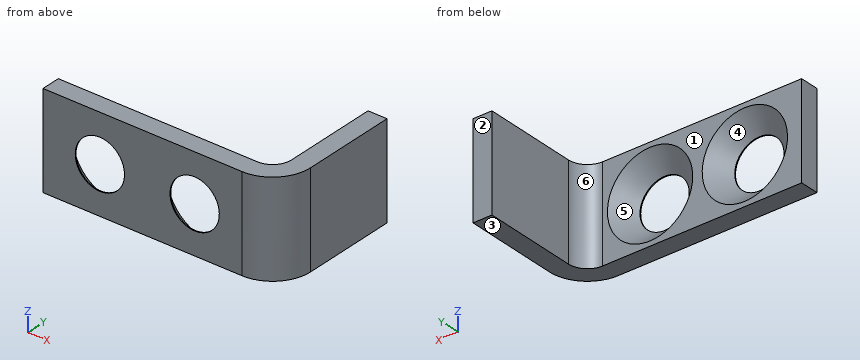
```python
from build123d import *

# Parameters (mm, degrees)
BASE_FLANGE1_DEPTH                          = 5
CSK_FOR_M2_CROSS_RECESSED_CTSK_HEAD_2_COUNT = 2
CSK_FOR_M2_CROSS_RECESSED_CTSK_HEAD_2_PITCH = 5


# Sheet-metal steps are written as plain solids
with BuildPart() as part:
    # Sketch1 → Base-Flange1 (new body)
    with BuildSketch(Plane.XY):
        with BuildLine():
            Line((-11.5, 0), (-1, 0))
            ThreePointArc((-1, 0), (-0.292893219, 0.292893219), (0, 1))
            Line((0, 1), (0, 6))
            Line((0, 6), (1, 6))
            Line((1, 6), (1, 1))
            ThreePointArc((1, 1), (0.414213562, -0.414213562), (-1, -1))
            Line((-1, -1), (-11.5, -1))
            Line((-11.5, -1), (-11.5, 0))
        make_face()
    extrude(amount=BASE_FLANGE1_DEPTH)

    # Sketch3 → CSK for M2 Cross recessed CTSK head wood screws1 (revolve, cut)
    with BuildSketch(Plane(origin=(-8.5, 0, 2.5), x_dir=(0, 0, 1), z_dir=(1, 0, 0))):
        Polygon((0, 0), (0, 1), (1.3, 1), (1.3, 0.95), (2.25, 0), align=None)
    csk_for_m2_cross_recessed_ctsk_head_wood = revolve(axis=Axis((-8.5, 6.35, 2.5), (0, -1, 0)), mode=Mode.SUBTRACT)

    # CSK for M2 Cross recessed CTSK head  2: CSK for M2 Cross recessed CTSK head wood screws1 ×2
    with Locations(*[(i * CSK_FOR_M2_CROSS_RECESSED_CTSK_HEAD_2_PITCH, 0, 0) for i in range(1, CSK_FOR_M2_CROSS_RECESSED_CTSK_HEAD_2_COUNT)]):
        add(csk_for_m2_cross_recessed_ctsk_head_wood, mode=Mode.SUBTRACT)


solid = part.part
```
The listing builds one solid part. Answer for the finished solid, in the listing's coordinates (mm). Face numbers are marked on the shaded views. A direction names the side the tool comes from. Give positions to 0.01 mm unless a question says otherwise; leave off trailing zeros. Loops run counter-clockwise (first coordinate to the right, second up) from the corner with the lowest first, then second, coordinate; pieces in that order, holes last. Notation, with made-up numbers: (24, 32) - (62, 32) arc R10 ccw to (62, 51) - close; hole circle Ø4 at (-29, 78.25). An arc over 180 degrees is marked (long way). Return JSON: item names as keys, results as strings. Group by question number.
1. Which of the six approach directions +Z, -Z, +X, -X, +Y, -Y give full straight-line access (tool end or side, diameter ignored) to the marked faces 1 and 2?
2. Straight lines are drawn through the part: line 1 (Y direction, x = -2.25, z = 0.4); line 2 (X direction, y = 1.5, z = 1.7); line 3 (Z direction, x = -9.5, y = -0.5). For each, find the intervals that lie inside material, in ascending order. Write a range as [from, to].
3. Find section B-B (y = -0.5). Write down the section's boundary in (x, z).
4. Find section C-C (z = 2.55). State how many separate pieces and enclosed holes the cut face has, then the cut area to 3 significant figures.
5. Find section A-A (x = -3.5). Write down the section's boundary in (y, z).
6. Determine the mould class of the marked faces 3, 4, 5 and 6 for opening direction Z: pulls with the +Z half, pulls with the -Z half, needs draft (parallel to the pull), parting line crosses it, or undercut.
7. Given pin 1 Ø2 at (y, z) = (2.5, 3.5) entering from -X; pin 2 Ø1.6 at (x, z) = (-8.5, 2.5) entering from -Y, each flat-ended and moving along its own axis, determine where each tip first touches the part or whether it passes through.
8. Find section D-D (y = 5.5). Write down the section's boundary in (x, z).
Verdict:
{
 "1": {"face 1": "+Z, -Z, -X, +Y", "face 2": "+Z, -Z, +X, -X, +Y"},
 "2": {"line 1": "y = [-1, 0]", "line 2": "x = [0, 1]", "line 3": "z = [0, 1.06], [3.94, 5]"},
 "3": {"outline": "(-11.5, 0) - (0.32, 0) - (0.32, 5) - (-11.5, 5) - close; hole circle Ø3.5 at (-8.5, 2.5); hole circle Ø3.5 at (-3.5, 2.5)"},
 "4": {"separate pieces": "3", "enclosed holes": "0", "area": "10.9 mm^2"},
 "5": {"outline": "(-1, 0) - (0, 0) - (0, 0.25) - (-0.95, 1.2) - (-1, 1.2) - close; (-1, 3.8) - (-0.95, 3.8) - (0, 4.75) - (0, 5) - (-1, 5) - close"},
 "6": {"face 3": "pulls with the -Z half", "face 4": "undercut", "face 5": "undercut", "face 6": "needs draft"},
 "7": {"pin 1": "stops at x = 0", "pin 2": "passes through"},
 "8": {"outline": "(0, 0) - (1, 0) - (1, 5) - (0, 5) - close"}
}
